Autodesk Inventor part; units mm, degrees
ref_plane "YZ Plane" through (0, 0, 0) normal (1, 0, 0) x (0, 1, 0)
ref_plane "XZ Plane" through (0, 0, 0) normal (0, 1, 0) x (-1, 0, 0)
ref_plane "XY Plane" through (0, 0, 0) normal (0, 0, 1) x (1, 0, 0)
sketch "Sketch1" plane through (0, 0, 0) normal (0, 1, 0) x (-1, 0, 0)
  line L0 (17.8, 24.25) -> (-17.8, 24.25)
  line L1 (-25.8, 16.25) -> (-25.8, -16.25)
  line L2 (-17.8, -24.25) -> (17.8, -24.25)
  line L3 (25.8, -16.25) -> (25.8, 16.25)
  line L4 (25.8, 24.25) -> (-25.8, -24.25) construction
  line L5 (-25.8, 24.25) -> (25.8, -24.25) construction
  line L6 (14, 24.25) -> (-14, 24.25)
  line L7 (-14, 24.25) -> (-14, 31.1)
  line L8 (-11, 34.1) -> (11, 34.1)
  line L9 (14, 31.1) -> (14, 24.25)
  line L10 (0, -38.0325) -> (0, 46.847)
  arc A0 (14, 31.1) -> (11, 34.1) centre (11, 31.1) ccw
  arc A1 (-11, 34.1) -> (-14, 31.1) centre (-11, 31.1) ccw
  arc A2 (17.8, -24.25) -> (25.8, -16.25) centre (17.8, -16.25) ccw
  arc A3 (-25.8, -16.25) -> (-17.8, -24.25) centre (-17.8, -16.25) ccw
  arc A4 (-17.8, 24.25) -> (-25.8, 16.25) centre (-17.8, 16.25) ccw
  arc A5 (25.8, 16.25) -> (17.8, 24.25) centre (17.8, 16.25) ccw
  point P0 (0, 0)
  point P1 (-14, 34.1)
  dimension "d0" = 48.5
  dimension "d1" = 51.6
  dimension "d2" = 9.85
  dimension "d3" = 28
  dimension "d5" = 3
  dimension "d10" = 8
extrude "Extrusion1" add sketch "Sketch1" along normal blind 5
shell "Shell1" thickness 1.5 removed faces 1 at (4.6667, 0, -8.0833)
sketch "Sketch2" plane through (0, 5, 0) normal (0, 1, 0) x (1, 0, 0)
  circle A0 centre (-9, -7.9) radius 1.05
  circle A1 centre (9, -7.9) radius 1.05
  circle A2 centre (-9, 7.9) radius 1.05
  circle A3 centre (9, 7.9) radius 1.05
  line L0 (-36.12, 0) -> (36.12, 0)
  line L1 (0, 35.92) -> (0, -45.77)
  circle A4 centre (-9, -26.9) radius 1.05
  circle A5 centre (9, -26.9) radius 1.05
  point P0 (0, 0)
  dimension "d11" = 2.1
  dimension "d12" = 18
  dimension "d13" = 15.8
  dimension "d14" = 19
extrude "Extrusion2" cut sketch "Sketch2" against normal through all
sketch "Sketch3" plane through (0, 5, 0) normal (0, 1, 0) x (1, 0, 0)
  circle A0 centre (9, -7.9) radius 1.05
  circle A1 centre (-9, 7.9) radius 1.05
  circle A2 centre (9, -26.9) radius 1.05
  circle A3 centre (-9, -7.9) radius 1.05
  circle A4 centre (9, 7.9) radius 1.05
  circle A5 centre (-9, -26.9) radius 1.05
  arc A6 (11, -34.1) -> (14, -31.1) centre (11, -31.1) ccw
  line L0 (11, -34.1) -> (-11, -34.1)
  arc A7 (-14, -31.1) -> (-11, -34.1) centre (-11, -31.1) ccw
  line L1 (-14, -31.1) -> (-14, -24.25)
  line L2 (-14, -24.25) -> (-17.8, -24.25)
  arc A8 (-25.8, -16.25) -> (-17.8, -24.25) centre (-17.8, -16.25) ccw
  line L3 (-25.8, -16.25) -> (-25.8, 16.25)
  arc A9 (-17.8, 24.25) -> (-25.8, 16.25) centre (-17.8, 16.25) ccw
  line L4 (-17.8, 24.25) -> (17.8, 24.25)
  arc A10 (25.8, 16.25) -> (17.8, 24.25) centre (17.8, 16.25) ccw
  line L5 (25.8, 16.25) -> (25.8, -16.25)
  arc A11 (17.8, -24.25) -> (25.8, -16.25) centre (17.8, -16.25) ccw
  line L6 (17.8, -24.25) -> (14, -24.25)
  line L7 (14, -24.25) -> (14, -31.1)
  line L8 (-24.3, 16.25) -> (-24.3, -16.25)
  arc A12 (-24.3, -16.25) -> (-17.8, -22.75) centre (-17.8, -16.25) ccw
  line L9 (-17.8, -22.75) -> (-12.5, -22.75)
  line L10 (-12.5, -22.75) -> (-12.5, -31.1)
  arc A13 (-12.5, -31.1) -> (-11, -32.6) centre (-11, -31.1) ccw
  line L11 (-11, -32.6) -> (11, -32.6)
  arc A14 (11, -32.6) -> (12.5, -31.1) centre (11, -31.1) ccw
  line L12 (12.5, -31.1) -> (12.5, -22.75)
  line L13 (12.5, -22.75) -> (17.8, -22.75)
  arc A15 (17.8, -22.75) -> (24.3, -16.25) centre (17.8, -16.25) ccw
  line L14 (24.3, -16.25) -> (24.3, 16.25)
  arc A16 (24.3, 16.25) -> (17.8, 22.75) centre (17.8, 16.25) ccw
  line L15 (17.8, 22.75) -> (-17.8, 22.75)
  arc A17 (-17.8, 22.75) -> (-24.3, 16.25) centre (-17.8, 16.25) ccw
  line L16 (-14, -24.25) -> (-14, -22.75)
  line L17 (14, -24.25) -> (14, -22.75)
  point P0 (0, 0)
  dimension "d17" = 1.5
extrude "Extrusion3" add sketch "Sketch3" along normal blind 1.6 contours L17 L13 A15 L14 A16 L15 A17 L8 A12 L9 L16 L2 A8 L3 A9 L4 A10 L5 A11 L6
sketch "Sketch4" plane through (0, 5, 0) normal (0, 1, 0) x (1, 0, 0)
  circle A0 centre (-9, 7.9) radius 2
  circle A1 centre (9, 7.9) radius 2
  circle A2 centre (9, -7.9) radius 2
  circle A3 centre (-9, -7.9) radius 2
  circle A4 centre (-9, -26.9) radius 2
  circle A5 centre (9, -26.9) radius 2
  circle A6 centre (9, 7.9) radius 1.05
  circle A7 centre (9, -7.9) radius 1.05
  circle A8 centre (9, -26.9) radius 1.05
  circle A9 centre (-9, -26.9) radius 1.05
  circle A10 centre (-9, -7.9) radius 1.05
  circle A11 centre (-9, 7.9) radius 1.05
  point P0 (0, 0)
  dimension "d20" = 4
extrude "Extrusion4" add sketch "Sketch4" along normal blind 1.6
sketch "Sketch5" plane through (0, 5, 0) normal (0, 1, 0) x (1, 0, 0)
  line L0 (-11, -34.1) -> (11, -34.1)
  line L1 (0, 38.0325) -> (0, -46.847)
  circle A0 centre (-9, 7.9) radius 1.05
  arc A1 (-14, -31.1) -> (-11, -34.1) centre (-11, -31.1) ccw
  circle A2 centre (9, -7.9) radius 2
  circle A3 centre (-9, 7.9) radius 2
  circle A4 centre (9, -26.9) radius 2
  circle A5 centre (-9, -7.9) radius 2
  circle A6 centre (9, 7.9) radius 2
  circle A7 centre (-9, -26.9) radius 2
  circle A8 centre (9, -7.9) radius 1.05
  circle A9 centre (-9, 7.9) radius 1.05
  circle A10 centre (9, -26.9) radius 1.05
  circle A11 centre (-9, -7.9) radius 1.05
  circle A12 centre (9, 7.9) radius 1.05
  circle A13 centre (-9, -26.9) radius 1.05
  line L2 (11, -34.1) -> (-11, -34.1)
  line L3 (-14, -31.1) -> (-14, -24.25)
  line L4 (-14, -22.75) -> (-14, -24.25)
  line L5 (-17.8, -22.75) -> (-14, -22.75)
  arc A14 (-24.3, -16.25) -> (-17.8, -22.75) centre (-17.8, -16.25) ccw
  line L6 (-24.3, 16.25) -> (-24.3, -16.25)
  arc A15 (-17.8, 22.75) -> (-24.3, 16.25) centre (-17.8, 16.25) ccw
  line L7 (17.8, 22.75) -> (-17.8, 22.75)
  arc A16 (24.3, 16.25) -> (17.8, 22.75) centre (17.8, 16.25) ccw
  line L8 (24.3, -16.25) -> (24.3, 16.25)
  arc A17 (17.8, -22.75) -> (24.3, -16.25) centre (17.8, -16.25) ccw
  line L9 (14, -22.75) -> (17.8, -22.75)
  line L10 (14, -24.25) -> (14, -22.75)
  line L11 (17.8, -24.25) -> (14, -24.25)
  arc A18 (17.8, -24.25) -> (25.8, -16.25) centre (17.8, -16.25) ccw
  line L12 (25.8, 16.25) -> (25.8, -16.25)
  arc A19 (25.8, 16.25) -> (17.8, 24.25) centre (17.8, 16.25) ccw
  line L13 (-17.8, 24.25) -> (17.8, 24.25)
  arc A20 (-17.8, 24.25) -> (-25.8, 16.25) centre (-17.8, 16.25) ccw
  line L14 (-25.8, -16.25) -> (-25.8, 16.25)
  arc A21 (-25.8, -16.25) -> (-17.8, -24.25) centre (-17.8, -16.25) ccw
  line L15 (-14, -24.25) -> (-17.8, -24.25)
  line L16 (14, -24.25) -> (14, -31.1)
  circle A22 centre (-9, -26.9) radius 3.5
  circle A23 centre (-9, -7.9) radius 3.5
  circle A24 centre (9, -7.9) radius 3.5
  circle A25 centre (9, -26.9) radius 3.5
  circle A26 centre (-9, 7.9) radius 2
  arc A27 (11, -34.1) -> (14, -31.1) centre (11, -31.1) ccw
  arc A28 (-14, -31.1) -> (-11, -34.1) centre (-11, -31.1) ccw
  line L17 (-11, 5.1) -> (11, 5.1)
  line L18 (14, 2.1) -> (14, -31.1)
  line L19 (11, -34.1) -> (-11, -34.1)
  line L20 (-14, -31.1) -> (-14, 2.1)
  arc A29 (-14, -31.1) -> (-11, -34.1) centre (-11, -31.1) ccw
  arc A30 (11, -34.1) -> (14, -31.1) centre (11, -31.1) ccw
  arc A31 (14, 2.1) -> (11, 5.1) centre (11, 2.1) ccw
  arc A32 (-11, 5.1) -> (-14, 2.1) centre (-11, 2.1) ccw
  point P0 (0, 0)
  point P1 (0, -34.1)
  point P2 (14, -24.2498)
  dimension "d25" = 7
  dimension "d30" = 39.2
extrude "Extrusion5" cut sketch "Sketch5" against normal blind 0.5 contours A1 L3 L4 L20 A32 L17 L1 L0 | L1 L17 A31 L18 L10 L16 A27 L0
properties part number "Pin-Base"
Can you work these out from the model? Positions are in its coordinate system, mm. A direction names the side the tool comes from. Coordinates: 2 decimals unless noted, no trailing zeros. Write each loop counter-clockwise with the first axis right and the second up, starting at its lowest first coordinate (ties: lowest second). Pieces come first, ordered by that corner, then holes. Notation, with made-up numbers: (-40, 85.5) -> (-19, 85.5) arc R20 ccw to (-19, 95.5) -> close; hole circle Ø9 at (83, 84.5). An arc over 180 degrees is marked (long way). Answer as CSV lines item,"result".
1) If we section it at D-D on z = 14: Please give me the cut outline in (x, y), then the cut area to 3 significant figures.
Check result:
outline,"(-25.8, 0) -> (-24.3, 0) -> (-24.3, 3.5) -> (24.3, 3.5) -> (24.3, 0) -> (25.8, 0) -> (25.8, 6.6) -> (24.3, 6.6) -> (24.3, 5) -> (14, 5) -> (14, 4.5) -> (-14, 4.5) -> (-14, 5) -> (-24.3, 5) -> (-24.3, 6.6) -> (-25.8, 6.6) -> close"
area,"78.7 mm²"
2) Will these pins go through, and if not, where does the flat tip stop? P1, Ø2.5, axis at x = -9, z = -7.9, coming from the -Y side; P2, Ø1.5, axis at y = 1, z = 25.5, coming from the -X side; P3, Ø1.1, axis at x = -16, y = 5, coming from the +Z side.
Check result:
P1,"y = 3.5"
P2,"x = -14"
P3,"z = 24.25"
3) If we section it at C-C on x = -4: Please give me the cut outline in (y, z).
Check result:
outline,"(0, -24.25) -> (6.6, -24.25) -> (6.6, -22.75) -> (5, -22.75) -> (5, -5.1) -> (4.5, -5.1) -> (4.5, 34.1) -> (0, 34.1) -> (0, 32.6) -> (3.5, 32.6) -> (3.5, -22.75) -> (0, -22.75) -> close"
4) If we section it at A-A on z = 26.9: Count the separate pieces of the cut face and the enclosed holes in it, then the cut area to 3 significant figures.
Check result:
separate pieces,"3"
enclosed holes,"0"
area,"45.3 mm²"
5) On a 3-axis mill with a long thin cutter (end or side, diameter ignored), from which of +Z, -Z, +X, -X, +Y, -Y can I reach the whole of each face in a straight line? I mean faces 5 (the cylindrical face through (22.345, 1.726, -20.896)), 6 (the cylindrical face through (23.519, 3.254, 21.844)), 7 (the cylindrical face through (-12.497, 4.754, 7.746)). Say none if no direction works.
Check result:
face 5,"-Y"
face 6,"+Z, +X, +Y, -Y"
face 7,"+Y"
6) If we mould it in two halves opening along X, with no side actions, what happens to faces 1 (the flat face through (14, 2, 28)), 2 (the flat face through (-16, 3, 24.25)), 3 (the flat face through (-24.3, 6, 0)), 4 (the flat face through (-11, 5, 6))? For each: +X half, -X half, draft (parallel to the pull), parting line (faces both ways), or undercut.
Check result:
face 1,"+X half"
face 2,"draft"
face 3,"undercut"
face 4,"undercut"
7) If we section it at B-B on y = 0.75: Please give me the cut outline in (x, z), then the cut area to 3 significant figures.
Check result:
outline,"(-25.8, -16.25) arc R8 ccw to (-17.8, -24.25) -> (17.8, -24.25) arc R8 ccw to (25.8, -16.25) -> (25.8, 16.25) arc R8 ccw to (17.8, 24.25) -> (14, 24.25) -> (14, 31.1) arc R3 ccw to (11, 34.1) -> (-11, 34.1) arc R3 ccw to (-14, 31.1) -> (-14, 24.25) -> (-17.8, 24.25) arc R8 ccw to (-25.8, 16.25) -> close; hole (-24.3, -16.25) arc R6.5 ccw to (-17.8, -22.75) -> (17.8, -22.75) arc R6.5 ccw to (24.3, -16.25) -> (24.3, 16.25) arc R6.5 ccw to (17.8, 22.75) -> (12.5, 22.75) -> (12.5, 31.1) arc R1.5 ccw to (11, 32.6) -> (-11, 32.6) arc R1.5 ccw to (-12.5, 31.1) -> (-12.5, 22.75) -> (-17.8, 22.75) arc R6.5 ccw to (-24.3, 16.25) -> close"
area,"299 mm²"
8) If I drill on line 1 (Z direction, x = -9, y = 4.4); line 2 (X direction, y = 5.2, z = -7.9); line 3 (X direction, y = 5.2, z = 26.9), over which ranges is the centre line in solid material (lowest first)? Write a range as from..to.
Check result:
line 1,"-24.25..-8.95, -6.85..6.85, 8.95..25.85, 27.95..34.1"
line 2,"-25.8..-24.3, -11..-10.05, -7.95..-7, 7..7.95, 10.05..11, 24.3..25.8"
line 3,"-11..-10.05, -7.95..-7, 7..7.95, 10.05..11"
